For this review, take the finished solid that the model builds, in its own axes (mm). Face numbers are marked on the shaded views. A direction names the side the tool comes from. Coordinates: 2 decimals unless noted, no trailing zeros. Write each loop counter-clockwise with the first axis right and the second up, starting at its lowest first coordinate (ties: lowest second). Pieces come first, ordered by that corner, then holes.
```python
from build123d import *

# Parameters (mm, degrees)
SKETCH1_W           = 10
SKETCH1_H           = 15
BOSS_EXTRUDE1_DEPTH = 10
SHELL1_T            = -1
BOSS_EXTRUDE4_REACH = 21.9
SKETCH5_W           = 9
SKETCH5_H           = 1
SKETCH3_R           = 0.5
BOSS_EXTRUDE3_DEPTH = 0.5
BOSS_EXTRUDE5_START = 0.5
SKETCH6_R           = 0.5
BOSS_EXTRUDE5_DEPTH = 0.5
SKETCH8_W           = 9
SKETCH8_H           = 13
CUT_EXTRUDE1_DEPTH  = 21.14944168
SKETCH10_W          = 1
SKETCH10_H          = 2
CUT_EXTRUDE4_DEPTH  = 9
FILLET1_R           = 1
FILLET2_R           = 1
FILLET3_R           = 1
FILLET5_R           = 1


with BuildPart() as part:
    # Sketch1 → Boss-Extrude1 (new body)
    with BuildSketch(Plane(origin=(0, 0, 0), x_dir=(1, 0, 0), z_dir=(0, 1, 0))):
        with Locations((5, 7.5)):
            Rectangle(SKETCH1_W, SKETCH1_H)
    extrude(amount=BOSS_EXTRUDE1_DEPTH)

    # Shell1
    shell1_openings = [part.faces().sort_by_distance(p)[0] for p in [
        (10, 5, -7.5),
    ]]
    offset(amount=SHELL1_T, openings=shell1_openings, kind=Kind.INTERSECTION)

    # Sketch5 → Boss-Extrude4 (add, up to next)
    with BuildSketch(Plane.XY.offset(-14), mode=Mode.PRIVATE) as boss_extrude4_sk1:
        with Locations((5.5, 6.5)):
            Rectangle(SKETCH5_W, SKETCH5_H)
    boss_extrude4_tool1 = extrude(boss_extrude4_sk1.sketch, amount=BOSS_EXTRUDE4_REACH, mode=Mode.PRIVATE) - part.part
    add(boss_extrude4_tool1.solids().sort_by_distance((5.5, 6.5, -14))[0])

    # Sketch3 → Boss-Extrude3 (add)
    with BuildSketch(Plane(origin=(0, 9, 0), x_dir=(-1, 0, 0), z_dir=(0, -1, 0))):
        with Locations(Location((-7.5, 2.5, 0), (0, 0, 90))):
            Circle(SKETCH3_R)
    extrude(amount=BOSS_EXTRUDE3_DEPTH)

    # Sketch6 → Boss-Extrude5 (add)
    with BuildSketch(Plane(origin=(0, 7, 0), x_dir=(1, 0, 0), z_dir=(0, 1, 0)).offset(BOSS_EXTRUDE5_START)):
        with Locations(Location((7.5, 2.5, 0), (0, 0, 90))):
            Circle(SKETCH6_R)
    extrude(amount=-BOSS_EXTRUDE5_DEPTH)

    # Sketch8 → Cut-Extrude1 (cut, through all)
    with BuildSketch(Plane(origin=(0, 1, 0), x_dir=(1, 0, 0), z_dir=(0, 1, 0))):
        with Locations((5.5, 7.5)):
            Rectangle(SKETCH8_W, SKETCH8_H)
    extrude(amount=-CUT_EXTRUDE1_DEPTH, mode=Mode.SUBTRACT)

    # Sketch10 → Cut-Extrude4 (cut)
    with BuildSketch(Plane(origin=(10, 0, 0), x_dir=(0, 0, -1), z_dir=(1, 0, 0))):
        with Locations((14.5, 8)):
            Rectangle(SKETCH10_W, SKETCH10_H)
    extrude(amount=-CUT_EXTRUDE4_DEPTH, mode=Mode.SUBTRACT)

    # Fillet1
    fillet1_edges = [part.edges().sort_by_distance(p)[0] for p in [
        (0, 10, -7.5),
        (0, 0, -7.5),
    ]]
    fillet(fillet1_edges, radius=FILLET1_R - 0.0001)  # a hair under: the kernel refuses the full size

    # Fillet2
    fillet2_edges = [part.edges().sort_by_distance(p)[0] for p in [
        (5.49995, 0, 0),
        (0.292863929, 0.292863929, 0),
        (0, 5, 0),
        (0.292863929, 9.707136071, 0),
        (5.49995, 10, 0),
    ]]
    fillet(fillet2_edges, radius=FILLET2_R - 0.0001)  # a hair under: the kernel refuses the full size

    # Fillet3
    fillet3_edges = [part.edges().sort_by_distance(p)[0] for p in [
        (5.49995, 0, -15),
        (0.292863929, 0.292863929, -15),
        (0, 5, -15),
        (0.292863929, 9.707136071, -15),
        (5.49995, 10, -15),
    ]]
    fillet(fillet3_edges, radius=FILLET3_R - 0.0001)  # a hair under: the kernel refuses the full size

    # Fillet5
    fillet5_edges = [part.edges().sort_by_distance(p)[0] for p in [
        (5.5, 6, -1),
        (5.5, 6, -14),
        (5.5, 7, -15),
    ]]
    fillet(fillet5_edges, radius=FILLET5_R)


solid = part.part
```
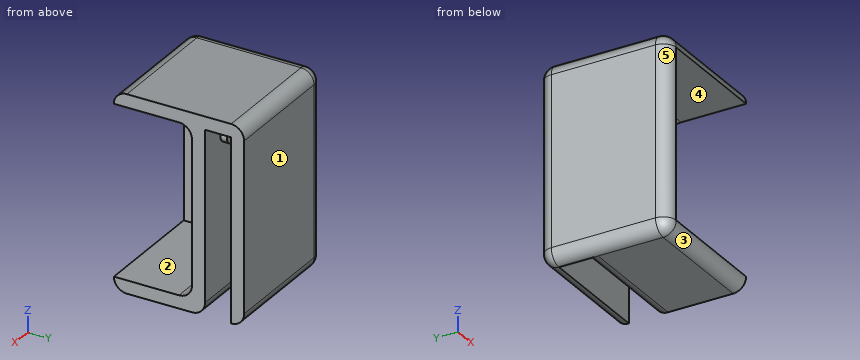
1) For L1, parallel to Z at x = 7, y = 4.25; L2, parallel to Y at x = 4.25, z = -2.25; L3, parallel to X at y = 8.25, z = -1.5, list the stretches that pass through material, from the lowest coordinate up.
2) Clearance check with flat-ended pins moving along their axes: P1, Ø1.5, axis at y = 8, z = -7.5, coming from the +X side; P2, Ø0.6, axis at x = 7.5, y = 8, coming from the -Z side; P3, Ø1, axis at x = 5, y = 7, coming from the -Z side. State where each tip first meets the part, or that it passes through.
3) The part is to be moulded in two halves that separate along Z. For the marked faces 3, 4 and 5, say which applies: pulls with the +Z half, pulls with the -Z half, needs draft (parallel to the pull), parting line crosses it, or undercut.
4) Consider section D-D (y = 4.5). Give the boundary of the cut face in (x, z), then the cut area to 3 significant figures.
5) Tool access review of the marked faces 1 and 2: name each direction out of +Z, -Z, +X, -X, +Y, -Y from which nothing blocks a thin tool from reaching the whole face with its end or side.
Results:
1. L1: z = -15 to -14, -1 to 0
1. L2: y = 6 to 7, 9 to 10
1. L3: x = 0 to 1
2. P1: stops at x = 1
2. P2: stops at z = -1
2. P3: stops at z = -14.87
3. face 3: pulls with the -Z half
3. face 4: undercut
3. face 5: needs draft
4. outline: (0, -14) arc R1 ccw to (1, -15) - (10, -15) - (10, -14) - (1, -14) - (1, -1) - (10, -1) - (10, 0) - (1, 0) arc R1 ccw to (0, -1) - close
4. area: 32.6 mm2
5. face 1: +Z, -Z, +X, -X, +Y
5. face 2: +X, -Y
